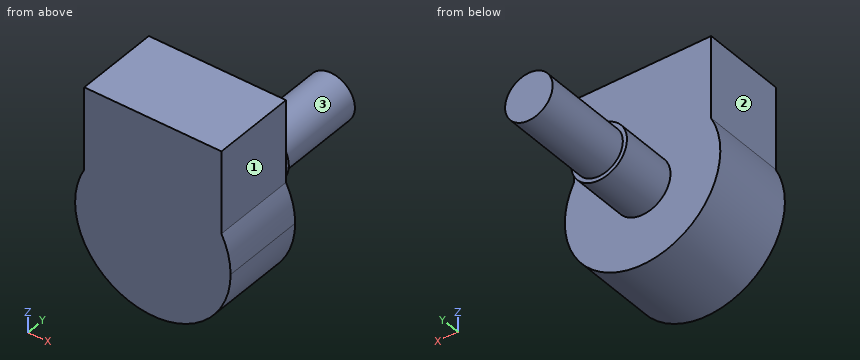
```python
from build123d import *

# Parameters (mm, degrees)
BOSS_EXTRUDE1_DEPTH = 9.2
SKETCH2_R           = 3.05
BOSS_EXTRUDE2_DEPTH = 6.2
SKETCH3_R           = 2.6
BOSS_EXTRUDE3_DEPTH = 10


with BuildPart() as part:
    # Sketch1 → Boss-Extrude1 (new body)
    with BuildSketch(Plane(origin=(0, 0, 0), x_dir=(1, 0, 0), z_dir=(0, 1, 0))):
        with BuildLine():
            ThreePointArc((8.5, 0), (-2.061552813, 8.246211251), (-7.5, -4))
            Line((-7.5, -4), (7.5, -4))
            ThreePointArc((7.5, -4), (8.246211251, -2.061552813), (8.5, 0))
        make_face()
        with BuildLine():
            Line((7.5, -4), (-7.5, -4))
            ThreePointArc((-7.5, -4), (0, -8.5), (7.5, -4))
        make_face()
        with BuildLine():
            ThreePointArc((7.5, -4), (0, -8.5), (-7.5, -4))
            Line((-7.5, -4), (-7.5, -13))
            Line((-7.5, -13), (7.5, -13))
            Line((7.5, -13), (7.5, -4))
        make_face()
    extrude(amount=BOSS_EXTRUDE1_DEPTH)

    # Sketch2 → Boss-Extrude2 (add)
    with BuildSketch(Plane(origin=(0, 9.2, 0), x_dir=(1, 0, 0), z_dir=(0, 1, 0))):
        with Locations(Location((0, 0, 0), (0, 0, 90))):
            Circle(SKETCH2_R)
    extrude(amount=BOSS_EXTRUDE2_DEPTH)

    # Sketch3 → Boss-Extrude3 (add)
    with BuildSketch(Plane(origin=(0, 15.4, 0), x_dir=(1, 0, 0), z_dir=(0, 1, 0))):
        with Locations(Location((0, 0, 0), (0, 0, 270))):
            Circle(SKETCH3_R)
    extrude(amount=BOSS_EXTRUDE3_DEPTH)


solid = part.part
```
Build history of the part. All positions in model axes, mm. Face numbers are marked on the shaded views. A direction names the side the tool comes from. Round coordinates to 2 decimals unless told otherwise and drop trailing zeros. Loops run counter-clockwise (first coordinate to the right, second up) from the corner with the lowest first, then second, coordinate; pieces in that order, holes last.
Item 1: Pin check, flat tips, straight feed: P1, Ø4, axis at y = 20.5, z = 3, coming from the +X side; P2, Ø5, axis at x = 4, z = 8.5, coming from the +Y side; P3, Ø1.5, axis at y = 6, z = 10.5, coming from the +X side. Stop position of each tip, or through.
Item 2: Drill centre lines: line 1 along Y through (x, z) = (-6.25, 9.5); line 2 along Z through (x, y) = (0.25, 9); line 3 along Z through (x, y) = (1.5, 16). Where is each one in solid material? Low to high.
Item 3: Saw through at C-C (z = 4.5). List the corners of the cut face in (x, y).
Item 4: Which spindle directions (+Z, -Z, +X, -X, +Y, -Y) get a long thin tool onto all of the face, cutting with end or side? Do the marked faces 1, 2 and 3. Say none if no direction does.
Item 5: Saw through at A-A (y = 2.75). List the corners of the cut face in (x, z), then the cut area to 3 significant figures.
Item 6: Saw through at D-D (y = 17.75). List the corners of the cut face in (x, z), then the cut area to 3 significant figures.
Item 7: Saw through at B-B (x = 0). List the corners of the cut face in (y, z), then the cut area to 3 significant figures.
Worked answers:
1. P1: stops at x = 2.4
1. P2: stops at y = 9.2
1. P3: stops at x = 7.5
2. line 1: y = 0 to 9.2
2. line 2: z = -8.5 to 13
2. line 3: z = -2.12 to 2.12
3. outline: (-7.5, 0) - (7.5, 0) - (7.5, 9.2) - (-7.5, 9.2) - close
4. face 1: +Z, +X, +Y, -Y
4. face 2: +Z, -X, +Y, -Y
4. face 3: +Y
5. outline: (-7.5, 4) arc R8.5 ccw (long way) to (7.5, 4) - (7.5, 13) - (-7.5, 13) - close
5. area: 314 mm2
6. outline: circle Ø5.2 at (0, 0)
6. area: 21.2 mm2
7. outline: (0, -8.5) - (9.2, -8.5) - (9.2, -3.05) - (15.4, -3.05) - (15.4, -2.6) - (25.4, -2.6) - (25.4, 2.6) - (15.4, 2.6) - (15.4, 3.05) - (9.2, 3.05) - (9.2, 13) - (0, 13) - close
7. area: 288 mm2
